Print and shaded views of the part. All mm, measured from the part's lowest x, y and z. Coordinates: 2 decimals unless noted, no trailing zeros. Order: outer loops, then holes, each group sorted by start corner. A loop starts at its lowest first (then second) coordinate and runs counter-clockwise, first axis right, second up. Notation, with made-up numbers: (41.25, 81.25) -> (96.25, 81.25) arc R25 cw to (96.25, 107.25) -> close; hole circle Ø7 at (-19, 0.5). An arc over 180 degrees is marked (long way). Return JSON: item names as keys, results as strings. Group by question number.
1) Flat gauge pin, fed straight in: pin 1 (1.5 mm diameter, centred on y = 9, z = 31, fed in from -X). Where does the tip first touch, or does it go through?
2) Cut at A-A (y = 8.75). Write the cut outline in (x, z), and give its area (3 significant figures).
3) Probe line 1 (Z direction, x = 90.5, y = 2.5) (1 decimal); line 2 (X direction, y = 1, z = 15.5) (1 decimal); line 3 (X direction, y = 8.75, z = 12.5) (1 decimal). List the from-to ranges inside material, lowest first.
4) Cut at B-B (z = 16). Write the cut outline in (x, y) (1 decimal), and give its area (3 significant figures).
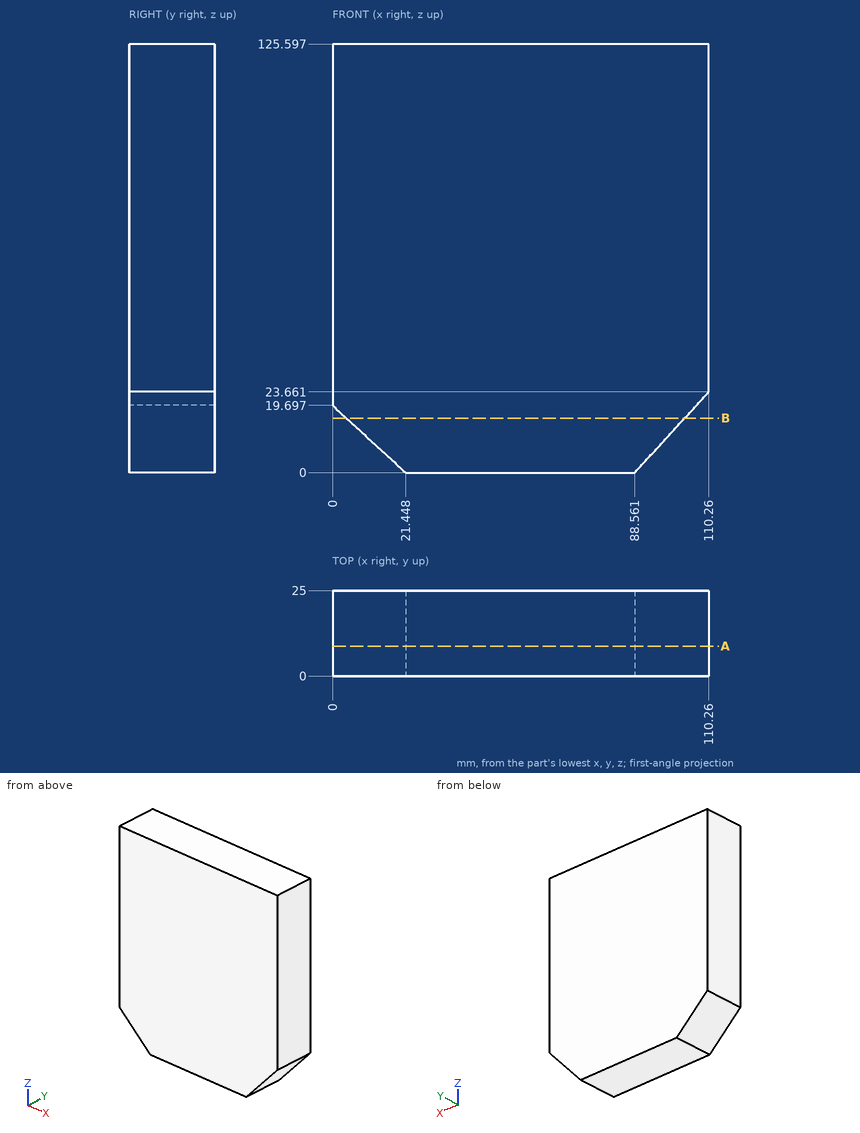
Answers below:
{
 "1": {"pin 1": "stops at x = 0"},
 "2": {"outline": "(0, 19.7) -> (21.45, 0) -> (88.56, 0) -> (110.26, 23.66) -> (110.26, 125.6) -> (0, 125.6) -> close", "area": "13,400 mm^2"},
 "3": {"line 1": "z = 2.1 to 125.6", "line 2": "x = 4.6 to 102.8", "line 3": "x = 7.8 to 100"},
 "4": {"outline": "(4, 0) -> (103.2, 0) -> (103.2, 25) -> (4, 25) -> close", "area": "2,480 mm^2"}
}
